Print and shaded views of the part. All mm, measured from the part's lowest x, y and z. Give positions to 0.01 mm unless a question says otherwise; leave off trailing zeros. Order: outer loops, then holes, each group sorted by start corner. A loop starts at its lowest first (then second) coordinate and runs counter-clockwise, first axis right, second up. Notation, with made-up numbers: (68, 10.25) - (124, 10.25) arc R11 ccw to (124, 29.25) - close; hole circle Ø1 at (79.25, -23). An arc over 180 degrees is marked (long way). Answer in a Markdown table with one row per item.
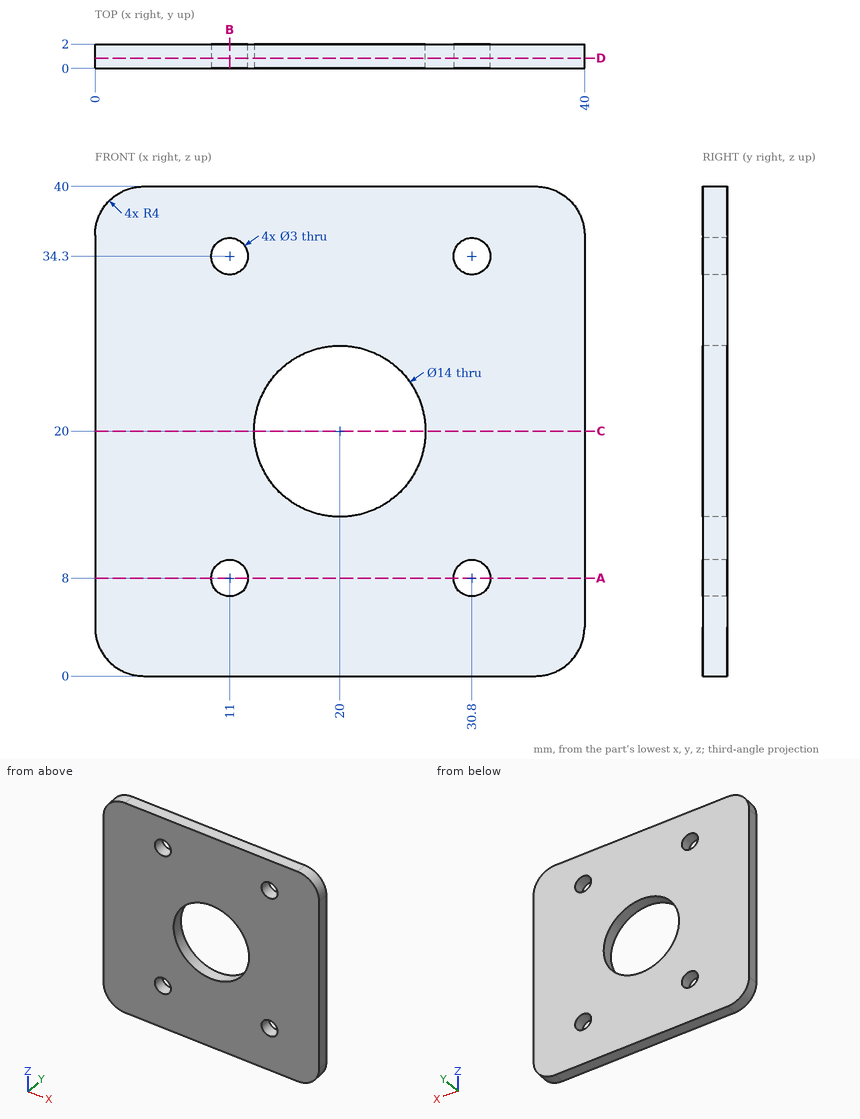
1. Drop a flat-ended pin along its axis: P1, Ø5, axis at x = 30.8, z = 8, coming from the +Y side. Give the stop position or say it passes through.
Check result:
| item | result |
|---|---|
| P1 | stops at y = 2 |
2. Cut at A-A on z = 8. Write the cut outline in (x, y), and give its area (3 significant figures).
Check result:
| item | result |
|---|---|
| outline | (0, 0) - (9.5, 0) - (9.5, 2) - (0, 2) - close; (12.5, 0) - (29.3, 0) - (29.3, 2) - (12.5, 2) - close; (32.3, 0) - (40, 0) - (40, 2) - (32.3, 2) - close |
| area | 68.0 mm² |
3. Probe line 1 (X direction, y = 1.35, z = 34.3); line 2 (Z direction, x = 11, y = 1.1); line 3 (X direction, y = 0.65, z = 20). List the from-to ranges inside material, lowest first.
Check result:
| item | result |
|---|---|
| line 1 | x = 0 to 9.5, 12.5 to 29.3, 32.3 to 40 |
| line 2 | z = 0 to 6.5, 9.5 to 32.8, 35.8 to 40 |
| line 3 | x = 0 to 13, 27 to 40 |
4. Cut at D-D on y = 0.85. Write the cut outline in (x, z).
Check result:
| item | result |
|---|---|
| outline | (0, 4) arc R4 ccw to (4, 0) - (36, 0) arc R4 ccw to (40, 4) - (40, 36) arc R4 ccw to (36, 40) - (4, 40) arc R4 ccw to (0, 36) - close; hole circle Ø3 at (11, 8); hole circle Ø3 at (11, 34.3); hole circle Ø14 at (20, 20); hole circle Ø3 at (30.8, 8); hole circle Ø3 at (30.8, 34.3) |
5. Cut at B-B on x = 11. Write the cut outline in (y, z).
Check result:
| item | result |
|---|---|
| outline | (0, 0) - (2, 0) - (2, 6.5) - (0, 6.5) - close; (0, 9.5) - (2, 9.5) - (2, 32.8) - (0, 32.8) - close; (0, 35.8) - (2, 35.8) - (2, 40) - (0, 40) - close |
6. Cut at C-C on z = 20. Write the cut outline in (x, y), and give its area (3 significant figures).
Check result:
| item | result |
|---|---|
| outline | (0, 0) - (13, 0) - (13, 2) - (0, 2) - close; (27, 0) - (40, 0) - (40, 2) - (27, 2) - close |
| area | 52.0 mm² |
